For this review, take the finished solid that the model builds, in its own axes (mm). Round coordinates to 2 decimals unless told otherwise and drop trailing zeros. Write each loop counter-clockwise with the first axis right and the second up, starting at its lowest first coordinate (ties: lowest second). Pieces come first, ordered by that corner, then holes. Notation, with made-up numbers: M 76,78.25 L 106,78.25 A33 ccw 106,109.25 Z; hole C 66,26.25 d5. An arc over 180 degrees is marked long. One line per question, with ' | ' between items.
```python
from build123d import *

# Parameters (mm, degrees)
F0_R     = 4.5
F1_DEPTH = 5
F2_SIZE  = 1
F3_SIZE  = 0.5


with BuildPart() as f1:
    # F0 (on Top) → F1 (new body)
    with BuildSketch(Plane.XY):
        with BuildLine():
            Line((55.8569601751, 37), (57.0526073024, 37))
            ThreePointArc((57.0526073024, 37), (0, 68), (-57.0526073024, 37))
            Line((-57.0526073024, 37), (-55.8569601751, 37))
            ThreePointArc((-55.8569601751, 37), (0, 67), (55.8569601751, 37))
        make_face()
        with BuildLine():
            Line((21.9089023002, 37), (55.8569601751, 37))
            ThreePointArc((55.8569601751, 37), (0, 67), (-55.8569601751, 37))
            Line((-55.8569601751, 37), (-21.9089023002, 37))
            ThreePointArc((-21.9089023002, 37), (0, 43), (21.9089023002, 37))
        make_face()
        with Locations((-27.5, 47.6313972081)):
            Circle(F0_R, mode=Mode.SUBTRACT)
        with BuildLine():
            Line((19.8746069144, 37), (21.9089023002, 37))
            ThreePointArc((21.9089023002, 37), (0, 43), (-21.9089023002, 37))
            Line((-21.9089023002, 37), (-19.8746069144, 37))
            ThreePointArc((-19.8746069144, 37), (0, 42), (19.8746069144, 37))
        make_face()
        with BuildLine():
            ThreePointArc((-21.9089023002, 37), (-25.438998692, 34.6678142598), (-28.7228132327, 32))
            Line((-28.7228132327, 32), (-27.2029410175, 32))
            ThreePointArc((-27.2029410175, 32), (-23.6711613534, 34.6940358013), (-19.8746069144, 37))
            Line((-19.8746069144, 37), (-21.9089023002, 37))
        make_face()
        with BuildLine():
            ThreePointArc((-55.8569601751, 37), (-57.4150594449, 34.5327518298), (-58.864250611, 32))
            Line((-58.864250611, 32), (-28.7228132327, 32))
            ThreePointArc((-28.7228132327, 32), (-25.438998692, 34.6678142598), (-21.9089023002, 37))
            Line((-21.9089023002, 37), (-55.8569601751, 37))
        make_face()
        with BuildLine():
            ThreePointArc((-57.0526073024, 37), (-58.579674112, 34.5314607413), (-60, 32))
            Line((-60, 32), (-58.864250611, 32))
            ThreePointArc((-58.864250611, 32), (-57.4150594449, 34.5327518298), (-55.8569601751, 37))
            Line((-55.8569601751, 37), (-57.0526073024, 37))
        make_face()
        with BuildLine():
            ThreePointArc((-58.864250611, 32), (-62.2890016221, 24.6795517974), (-64.8074069841, 17))
            Line((-64.8074069841, 17), (-39.4968353163, 17))
            ThreePointArc((-39.4968353163, 17), (-34.9246347445, 25.0852523999), (-28.7228132327, 32))
            Line((-28.7228132327, 32), (-58.864250611, 32))
        make_face()
        with BuildLine():
            ThreePointArc((-60, 32), (-63.3657755146, 24.6734370008), (-65.8407168855, 17))
            Line((-65.8407168855, 17), (-64.8074069841, 17))
            ThreePointArc((-64.8074069841, 17), (-62.2890016221, 24.6795517974), (-58.864250611, 32))
            Line((-58.864250611, 32), (-60, 32))
        make_face()
        with BuildLine():
            ThreePointArc((-28.7228132327, 32), (-34.9246347445, 25.0852523999), (-39.4968353163, 17))
            Line((-39.4968353163, 17), (-38.4057287393, 17))
            ThreePointArc((-38.4057287393, 17), (-33.6507709691, 25.1321629229), (-27.2029410175, 32))
            Line((-27.2029410175, 32), (-28.7228132327, 32))
        make_face()
        with BuildLine():
            Line((39.4968353163, 17), (64.8074069841, 17))
            ThreePointArc((64.8074069841, 17), (62.2890016221, 24.6795517974), (58.864250611, 32))
            Line((58.864250611, 32), (28.7228132327, 32))
            ThreePointArc((28.7228132327, 32), (34.9246347445, 25.0852523999), (39.4968353163, 17))
        make_face()
        with BuildLine():
            Line((58.864250611, 32), (60, 32))
            ThreePointArc((60, 32), (58.579674112, 34.5314607413), (57.0526073024, 37))
            Line((57.0526073024, 37), (55.8569601751, 37))
            ThreePointArc((55.8569601751, 37), (57.4150594449, 34.5327518298), (58.864250611, 32))
        make_face()
        with BuildLine():
            Line((28.7228132327, 32), (58.864250611, 32))
            ThreePointArc((58.864250611, 32), (57.4150594449, 34.5327518298), (55.8569601751, 37))
            Line((55.8569601751, 37), (21.9089023002, 37))
            ThreePointArc((21.9089023002, 37), (25.438998692, 34.6678142598), (28.7228132327, 32))
        make_face()
        with BuildLine():
            Line((27.2029410175, 32), (28.7228132327, 32))
            ThreePointArc((28.7228132327, 32), (25.438998692, 34.6678142598), (21.9089023002, 37))
            Line((21.9089023002, 37), (19.8746069144, 37))
            ThreePointArc((19.8746069144, 37), (23.6711613534, 34.6940358013), (27.2029410175, 32))
        make_face()
        with BuildLine():
            Line((38.4057287393, 17), (39.4968353163, 17))
            ThreePointArc((39.4968353163, 17), (34.9246347445, 25.0852523999), (28.7228132327, 32))
            Line((28.7228132327, 32), (27.2029410175, 32))
            ThreePointArc((27.2029410175, 32), (33.6507709691, 25.1321629229), (38.4057287393, 17))
        make_face()
        with BuildLine():
            Line((64.8074069841, 17), (65.8407168855, 17))
            ThreePointArc((65.8407168855, 17), (63.3657755146, 24.6734370008), (60, 32))
            Line((60, 32), (58.864250611, 32))
            ThreePointArc((58.864250611, 32), (62.2890016221, 24.6795517974), (64.8074069841, 17))
        make_face()
        with BuildLine():
            Line((65.9166139907, 12), (66.9328021227, 12))
            ThreePointArc((66.9328021227, 12), (66.4338154667, 14.5102778244), (65.8407168855, 17))
            Line((65.8407168855, 17), (64.8074069841, 17))
            ThreePointArc((64.8074069841, 17), (65.4098036609, 14.5106025046), (65.9166139907, 12))
        make_face()
        with BuildLine():
            Line((41.2916456441, 12), (65.9166139907, 12))
            ThreePointArc((65.9166139907, 12), (65.4098036609, 14.5106025046), (64.8074069841, 17))
            Line((64.8074069841, 17), (39.4968353163, 17))
            ThreePointArc((39.4968353163, 17), (40.471529054, 14.5277436661), (41.2916456441, 12))
        make_face()
        with BuildLine():
            Line((40.249223595, 12), (41.2916456441, 12))
            ThreePointArc((41.2916456441, 12), (40.471529054, 14.5277436661), (39.4968353163, 17))
            Line((39.4968353163, 17), (38.4057287393, 17))
            ThreePointArc((38.4057287393, 17), (39.4068570388, 14.5292676457), (40.249223595, 12))
        make_face()
        with BuildLine():
            ThreePointArc((43, 0), (42.5707690951, 6.060496568), (41.2916456441, 12))
            Line((41.2916456441, 12), (40.249223595, 12))
            ThreePointArc((40.249223595, 12), (41.5600011489, 6.0635224503), (42, 0))
            ThreePointArc((42, 0), (-6.0635224503, -41.5600011489), (-40.249223595, 12))
            Line((-40.249223595, 12), (-41.2916456441, 12))
            ThreePointArc((-41.2916456441, 12), (-6.060496568, -42.5707690951), (43, 0))
        make_face()
        with BuildLine():
            ThreePointArc((67, 0), (66.7286038269, 6.0244029838), (65.9166139907, 12))
            Line((65.9166139907, 12), (41.2916456441, 12))
            ThreePointArc((41.2916456441, 12), (42.5707690951, 6.060496568), (43, 0))
            ThreePointArc((43, 0), (-6.060496568, -42.5707690951), (-41.2916456441, 12))
            Line((-41.2916456441, 12), (-65.9166139907, 12))
            ThreePointArc((-65.9166139907, 12), (-6.0244029838, -66.7286038269), (67, 0))
        make_face()
        with Locations((-27.5, -47.6313972081)):
            Circle(F0_R, mode=Mode.SUBTRACT)
        with Locations((55, 0)):
            Circle(F0_R, mode=Mode.SUBTRACT)
        with BuildLine():
            ThreePointArc((-66.9328021227, 12), (-6.0236805881, -67.7326750703), (68, 0))
            ThreePointArc((68, 0), (67.7326750703, 6.0236805881), (66.9328021227, 12))
            Line((66.9328021227, 12), (65.9166139907, 12))
            ThreePointArc((65.9166139907, 12), (66.7286038269, 6.0244029838), (67, 0))
            ThreePointArc((67, 0), (-6.0244029838, -66.7286038269), (-65.9166139907, 12))
            Line((-65.9166139907, 12), (-66.9328021227, 12))
        make_face()
        with BuildLine():
            ThreePointArc((-39.4968353163, 17), (-40.471529054, 14.5277436661), (-41.2916456441, 12))
            Line((-41.2916456441, 12), (-40.249223595, 12))
            ThreePointArc((-40.249223595, 12), (-39.4068570388, 14.5292676457), (-38.4057287393, 17))
            Line((-38.4057287393, 17), (-39.4968353163, 17))
        make_face()
        with BuildLine():
            ThreePointArc((-65.8407168855, 17), (-66.4338154667, 14.5102778244), (-66.9328021227, 12))
            Line((-66.9328021227, 12), (-65.9166139907, 12))
            ThreePointArc((-65.9166139907, 12), (-65.4098036609, 14.5106025046), (-64.8074069841, 17))
            Line((-64.8074069841, 17), (-65.8407168855, 17))
        make_face()
        with BuildLine():
            ThreePointArc((-64.8074069841, 17), (-65.4098036609, 14.5106025046), (-65.9166139907, 12))
            Line((-65.9166139907, 12), (-41.2916456441, 12))
            ThreePointArc((-41.2916456441, 12), (-40.471529054, 14.5277436661), (-39.4968353163, 17))
            Line((-39.4968353163, 17), (-64.8074069841, 17))
        make_face()
    extrude(amount=F1_DEPTH)

    # F2
    f2_edges = [f1.edges().sort_by_distance(p)[0] for p in [
        (65.840717, -17, 5),
        (40.249224, -12, 5),
    ]]
    chamfer(f2_edges, length=F2_SIZE)

    # F3
    f3_edges = [f1.edges().sort_by_distance(p)[0] for p in [
        (-32, 47.631397, 5),
        (40.249224, -12, 0),
        (-32, 47.631397, 0),
        (65.840717, -17, 0),
        (50.5, 0, 5),
        (50.5, 0, 0),
        (-32, -47.631397, 5),
        (-32, -47.631397, 0),
    ]]
    chamfer(f3_edges, length=F3_SIZE)


solid = f1.part
```
Item 1: To check wall thickness, follow line 1 along Y through (x, z) = (0, 2.45); line 2 along X through (y, z) = (8, 0.6); line 3 along Y through (x, z) = (5.5, 4.75). State the ranges of each line that lie inside material, in increasing order. Write a range as from..to.
Results:
line 1: -68..-42, 42..68 | line 2: -67.53..-41.23, 41.23..67.53 | line 3: -67.02..-42.39, 42.39..67.02
Item 2: Mouldability with a two-part tool opening along X and no side actions: class faces 1 (the face through (-25.081, 51.426, 2.472)), 2 (the face through (-1, -44, 5)) as +X half, -X half, draft (parallel to the pull), parting line (faces both ways), or undercut.
Results:
face 1: undercut | face 2: draft
Item 3: Insertion check: pin 1 Ø3 at (x, z) = (-6, 4) entering from -Y; pin 2 Ø2 at (x, z) = (33.5, 3) entering from +Y; pin 3 Ø2 at (y, z) = (37, 1) entering from -X. Each pin has a flat end and moves straight along its axis. Give the tip position at first contact, or say it passes through.
Results:
pin 1: y = -67.85 | pin 2: y = 59.73 | pin 3: x = -57.69
Item 4: Take a section at A-A (x = 0). Write out the cut boundary in (y, z), then the cut area to 4 significant figures.
Results:
outline: M -68,0.5 L -67.5,0 L -42.5,0 L -42,0.5 L -42,4 L -43,5 L -67,5 L -68,4 Z; M 42,0.5 L 42.5,0 L 67.5,0 L 68,0.5 L 68,4 L 67,5 L 43,5 L 42,4 Z | area: 257.5 mm2
